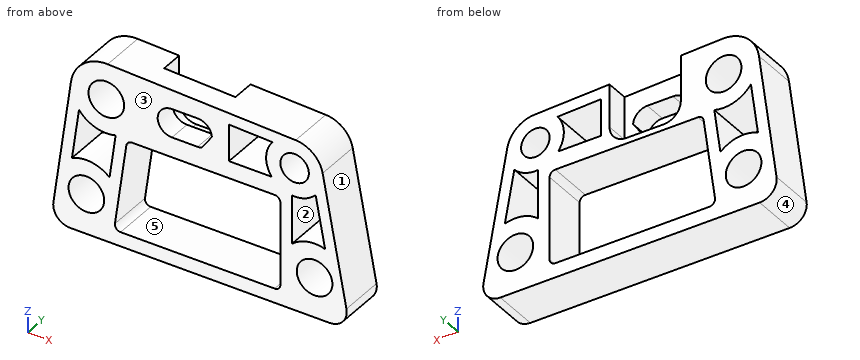
```python
from build123d import *

# Parameters (mm, degrees)
SKETCH3_R           = 3.96875
SKETCH3_R_2         = 3.175
BOSS_EXTRUDE4_DEPTH = 10.16
CUT_EXTRUDE3_DEPTH  = 5.08
FILLET1_R           = 3.81


with BuildPart() as part:
    # Sketch3 → Boss-Extrude4 (new body)
    with BuildSketch(Plane(origin=(0, 0, 0), x_dir=(1, 0, 0), z_dir=(0, 1, 0))):
        with BuildLine():
            Line((54.2925, 31.75), (-12.3825, 31.75))
            Line((-12.3825, 31.75), (-7.863361559, -1.082336008))
            ThreePointArc((-7.863361559, -1.082336008), (-5.101706023, -6.080830692), (0.300662879, -7.931803583))
            Line((0.300662879, -7.931803583), (42.150530303, -6.345442867))
            ThreePointArc((42.150530303, -6.345442867), (46.059378881, -4.806782177), (48.152310263, -1.164501002))
            Line((48.152310263, -1.164501002), (54.2925, 31.75))
        make_face()
        with Locations(Location((0, 0, 0), (0, 0, 270))):
            Circle(SKETCH3_R, mode=Mode.SUBTRACT)
        with Locations(Location((-4.445, 22.86, 0), (0, 0, 270))):
            Circle(SKETCH3_R, mode=Mode.SUBTRACT)
        with Locations(Location((46.355, 22.86, 0), (0, 0, 270))):
            Circle(SKETCH3_R, mode=Mode.SUBTRACT)
        with Locations(Location((41.91, 0, 0), (0, 0, 270))):
            Circle(SKETCH3_R_2, mode=Mode.SUBTRACT)
        with BuildLine():
            Line((38.735, 8.89), (38.735, 27.305))
            ThreePointArc((38.735, 27.305), (38.363025612, 28.203025612), (37.465, 28.575))
            Line((37.465, 28.575), (3.175, 28.575))
            ThreePointArc((3.175, 28.575), (2.217704153, 28.139556566), (1.91686215, 27.131826239))
            Line((1.91686215, 27.131826239), (4.451556434, 8.716826239))
            ThreePointArc((4.451556434, 8.716826239), (4.875137717, 7.932704153), (5.709694283, 7.62))
            Line((5.709694283, 7.62), (37.465, 7.62))
            ThreePointArc((37.465, 7.62), (38.363025612, 7.991974388), (38.735, 8.89))
        make_face(mode=Mode.SUBTRACT)
        with BuildLine():
            Line((20.32, 3.175), (14.605, 3.175))
            ThreePointArc((14.605, 3.175), (11.43, 0), (14.605, -3.175))
            Line((14.605, -3.175), (20.32, -3.175))
            ThreePointArc((20.32, -3.175), (22.498043553, -2.310140965), (23.489504023, -0.186733089))
            Line((23.489504023, -0.186733089), (21.228562514, 3.04222602))
            ThreePointArc((21.228562514, 3.04222602), (20.779106407, 3.141631154), (20.32, 3.175))
        make_face(mode=Mode.SUBTRACT)
        with BuildLine():
            Line((46.58698696, 4.295147609), (48.697586564, 15.60902157))
            ThreePointArc((48.697586564, 15.60902157), (44.776818872, 15.405220035), (41.275, 17.180387337))
            Line((41.275, 17.180387337), (41.275, 6.318170226))
            ThreePointArc((41.275, 6.318170226), (44.169993312, 5.934216901), (46.58698696, 4.295147609))
        make_face(mode=Mode.SUBTRACT)
        with BuildLine():
            Line((-6.080523252, 4.592563226), (-7.642900683, 15.943510195))
            ThreePointArc((-7.642900683, 15.943510195), (-3.266927549, 15.331617352), (0.712930912, 17.251065278))
            Line((0.712930912, 17.251065278), (2.078345222, 7.331090037))
            ThreePointArc((2.078345222, 7.331090037), (-2.424714317, 7.223929712), (-6.080523252, 4.592563226))
        make_face(mode=Mode.SUBTRACT)
        with BuildLine():
            Line((36.977963889, -3.999689962), (27.305, -4.366353249))
            Line((27.305, -4.366353249), (27.305, 3.81))
            Line((27.305, 3.81), (36.83, 3.81))
            ThreePointArc((36.83, 3.81), (35.561139386, -0.120286735), (36.977963889, -3.999689962))
        make_face(mode=Mode.SUBTRACT)
    extrude(amount=BOSS_EXTRUDE4_DEPTH)

    # Sketch5 → Cut-Extrude3 (cut)
    with BuildSketch(Plane(origin=(0, 10.16, 0), x_dir=(1, 0, 0), z_dir=(0, 1, 0))):
        with BuildLine():
            Line((25.4, 2.577854061), (25.4, -7.582145939))
            Line((25.4, -7.582145939), (9.525, -7.582145939))
            Line((9.525, -7.582145939), (9.525, 2.577854061))
            ThreePointArc((9.525, 2.577854061), (10.640923164, 5.271930897), (13.335, 6.387854061))
            Line((13.335, 6.387854061), (21.59, 6.387854061))
            ThreePointArc((21.59, 6.387854061), (24.284076836, 5.271930897), (25.4, 2.577854061))
        make_face()
    extrude(amount=-CUT_EXTRUDE3_DEPTH, mode=Mode.SUBTRACT)

    # Fillet1
    fillet1_edges = [part.edges().sort_by_distance(p)[0] for p in [
        (-12.3825, 5.08, -31.75),
        (54.2925, 5.08, -31.75),
    ]]
    fillet(fillet1_edges, radius=FILLET1_R)


solid = part.part
```
Work out the finished part from the listing and answer in its coordinate system (mm). Face numbers are marked on the shaded views. A direction names the side the tool comes from. Coordinates: 2 decimals unless noted, no trailing zeros. Write each loop counter-clockwise with the first axis right and the second up, starting at its lowest first coordinate (ties: lowest second). Pieces come first, ordered by that corner, then holes.
Q1. A cutting plane is placed at A-A, the plane z = -12.5. Give the vertices of the cut face in (x, y) (3 decimals), then the cut area to 3 significant figures.
Q2. Determine the mould class of the marked faces 3, 4 and 5 for opening direction X: released by +X, released by -X, zero draft, split by the parting line, or undercut.
Q3. A cutting plane is placed at B-B, the plane z = -0.5. Give the vertices of the cut face in (x, y) (3 decimals), then the cut area to 3 significant figures.
Q4. A cutting plane is placed at C-C, the plane z = -22.86. Give the vertices of the cut face in (x, y) (3 decimals), then the cut area to 3 significant figures.
Q5. Each of these flat-tipped pins is pushed along its axis until it touches: pin 1 Ø5.5 at (x, y) = (16.5, 7.5) entering from +Z; pin 2 Ø4 at (y, z) = (6, 2) entering from +X; pin 3 Ø2.5 at (x, y) = (18.5, 3.5) entering from +Z. Where does it stop, or does it pass through?
Q6. Find the intervals of material crossed by line 1 (X direction, y = 1.25, z = 1) (3 decimals); line 2 (X direction, y = 7.25, z = -25) (3 decimals); line 3 (X direction, y = 5.25, z = 0) (3 decimals), in increasing order.
Q7. Which of the six approach directions +Z, -Z, +X, -X, +Y, -Y give full straight-line access (tool end or side, diameter ignored) to the marked faces 1 and 2?
Q8. A cutting plane is placed at D-D, the plane y = 1.25. State how many separate pieces and enclosed holes the cut face has, then the cut area to 3 significant figures.
Findings below:
1. outline: (-9.733, 0) - (-7.169, 0) - (-7.169, 10.16) - (-9.733, 10.16) - close; (1.367, 0) - (3.931, 0) - (3.931, 10.16) - (1.367, 10.16) - close; (38.735, 0) - (41.275, 0) - (41.275, 10.16) - (38.735, 10.16) - close; (48.118, 0) - (50.701, 0) - (50.701, 10.16) - (48.118, 10.16) - close
1. area: 104 mm2
2. face 3: zero draft
2. face 4: released by -X
2. face 5: undercut
3. outline: (-8.081, 0) - (-3.937, 0) - (-3.937, 10.16) - (-8.081, 10.16) - close; (3.937, 0) - (11.47, 0) - (11.47, 5.08) - (9.525, 5.08) - (9.525, 10.16) - (3.937, 10.16) - close; (23.009, 0) - (27.305, 0) - (27.305, 10.16) - (25.4, 10.16) - (25.4, 5.08) - (23.009, 5.08) - close; (35.58, 0) - (38.775, 0) - (38.775, 10.16) - (35.58, 10.16) - close; (45.045, 0) - (48.463, 0) - (48.463, 10.16) - (45.045, 10.16) - close
3. area: 207 mm2
4. outline: (-11.159, 0) - (-8.414, 0) - (-8.414, 10.16) - (-11.159, 10.16) - close; (-0.476, 0) - (2.505, 0) - (2.505, 10.16) - (-0.476, 10.16) - close; (38.735, 0) - (42.386, 0) - (42.386, 10.16) - (38.735, 10.16) - close; (50.324, 0) - (52.634, 0) - (52.634, 10.16) - (50.324, 10.16) - close
4. area: 119 mm2
5. pin 1: stops at z = 7.37
5. pin 2: stops at x = 48.37
5. pin 3: stops at z = 7.29
6. line 1: x = -7.875 to -3.841, 3.841 to 11.592, 23.333 to 27.305, 35.639 to 38.897, 44.923 to 48.183
6. line 2: x = -11.453 to -7.787, -1.103 to 2.21, 38.735 to 43.013, 49.697 to 53.033
6. line 3: x = -8.012 to -3.969, 3.969 to 9.525, 25.4 to 27.305, 35.56 to 38.735, 45.085 to 48.37
7. face 1: +Z, +X, +Y, -Y
7. face 2: +Y, -Y
8. separate pieces: 1
8. enclosed holes: 9
8. area: 1,130 mm2
